Geometry: see drawing. Coordinates: mm, zero at the bounding-box minimum. A direction names the side the tool comes from. Give positions to 0.01 mm unless a question says otherwise; leave off trailing zeros. Write each loop counter-clockwise with the first axis right and the second up, starting at its lowest first coordinate (ties: lowest second). Pieces come first, ordered by that corner, then holes. Notation, with made-up numbers: M -2.75,86 L 48.25,86 A22 ccw 48.25,124 Z; hole C 55,53 d9. An arc over 180 degrees is marked long. Use a Markdown table: item, result. Add a question column.
(1) Cut plane C-C (z = 76). Output: boundary loops of the cut face in (x, y), plus the area to 3 significant figures.
(2) Draft query along Z for the marked faces 1, 2, 3 and 4. Return one class per face: released by +Z, released by -Z, zero draft, split by the parting line, or undercut.
(3) Cut plane D-D (x = 49.5). Output: boundary loops of the cut face in (y, z), plus the area to 3 significant figures.
(4) Reachability of the marked faces 5 and 6 from +Z, -Z, +X, -X, +Y, -Y: full face, straight path, thin tool, end or side. Return the list, or none.
(5) Material intervals for L1, parallel to Z at x = 177, y = 57; L2, parallel to X at y = 87, z = 31.5; L3, parallel to Y at x = 185, z = 97.7, sorted ascending.
(6) Cut plane A-A (y = 70). Output: boundary loops of the cut face in (x, z), plus the area to 3 significant figures.
(7) Pin query (flat end, axial travel): pin 1 Ø2 at (x, z) = (112.5, 50.5) entering from +Y; pin 2 Ø4.5 at (x, y) = (185, 70) entering from +Z. Return the tip coordinate at first contact, or that it passes through.
(8) Cut plane B-B (x = 185). Output: boundary loops of the cut face in (y, z).
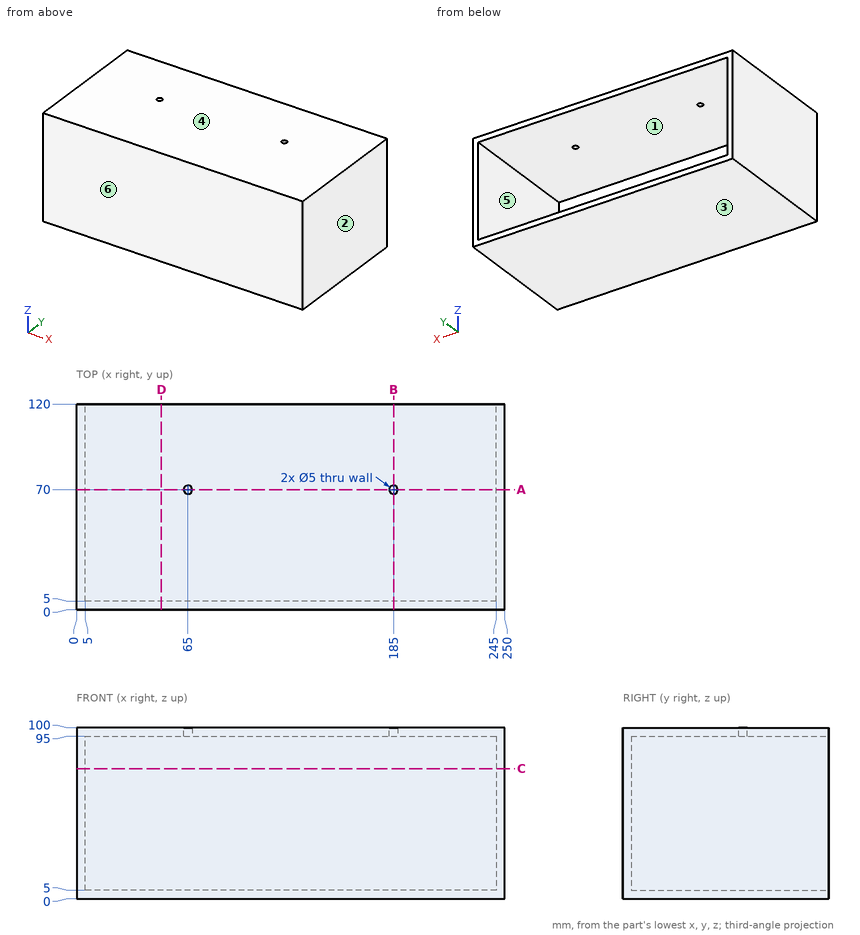
Answer list:
| question | item | result |
|---|---|---|
| 1 | outline | M 0,0 L 250,0 L 250,120 L 245,120 L 245,5 L 5,5 L 5,120 L 0,120 Z |
| 1 | area | 2,400 mm² |
| 2 | face 1 | undercut |
| 2 | face 2 | zero draft |
| 2 | face 3 | released by -Z |
| 2 | face 4 | released by +Z |
| 3 | outline | M 0,0 L 120,0 L 120,5 L 5,5 L 5,95 L 120,95 L 120,100 L 0,100 Z |
| 3 | area | 1,650 mm² |
| 4 | face 5 | +Y |
| 4 | face 6 | +Z, -Z, +X, -X, -Y |
| 5 | L1 | 0 to 5, 95 to 100 |
| 5 | L2 | 0 to 5, 245 to 250 |
| 5 | L3 | 0 to 67.5, 72.5 to 120 |
| 6 | outline | M 0,0 L 250,0 L 250,100 L 187.5,100 L 187.5,95 L 245,95 L 245,5 L 5,5 L 5,95 L 62.5,95 L 62.5,100 L 0,100 Z; M 67.5,95 L 182.5,95 L 182.5,100 L 67.5,100 Z |
| 6 | area | 3,350 mm² |
| 7 | pin 1 | y = 5 |
| 7 | pin 2 | z = 5 |
| 8 | outline | M 0,0 L 120,0 L 120,5 L 5,5 L 5,95 L 67.5,95 L 67.5,100 L 0,100 Z; M 72.5,95 L 120,95 L 120,100 L 72.5,100 Z |
